```python
from build123d import *

# Parameters (mm, degrees)
SKETCH1_W               = 51
SKETCH1_H               = 26
PCB_DEPTH               = 1.6
MOUNT_HOLE_1_DEPTH      = 58.267442758
MOUNT_HOLE_1_DEPTH_BACK = 58.267442758
SKETCH2_R               = 1.5
MOUNT_HOLE_2_DEPTH      = 58.267442758
MOUNT_HOLE_2_DEPTH_BACK = 58.267442758
SKETCH3_R               = 1.5
MOUNT_HOLE_3_DEPTH      = 58.267442758
MOUNT_HOLE_3_DEPTH_BACK = 58.267442758
SKETCH4_R               = 1.5
MOUNT_HOLE_4_DEPTH      = 58.267442758
MOUNT_HOLE_4_DEPTH_BACK = 58.267442758
SKETCH5_R               = 1.5
INDUCTOR_START          = 1.6
SKETCH6_W               = 14
SKETCH6_H               = 14
INDUCTOR_DEPTH          = 8
CAP_IN_START            = 1.6
SKETCH7_R               = 5
CAP_IN_DEPTH            = 13
CAP_OUT_START           = 1.6
SKETCH8_R               = 5
CAP_OUT_DEPTH           = 13
HEATSINK_START          = 1.6
SKETCH9_W               = 8
SKETCH9_H               = 16
HEATSINK_DEPTH          = 11
TRIM_POT_START          = 1.6
SKETCH10_W              = 9.5
SKETCH10_H              = 4.5
TRIM_POT_DEPTH          = 9.5


with BuildPart() as part:
    # Sketch1 → PCB (new body)
    with BuildSketch(Plane(origin=(0, 0, 0), x_dir=(1, 0, 0), z_dir=(0, 1, 0))):
        with Locations((25.5, 13)):
            Rectangle(SKETCH1_W, SKETCH1_H)
    extrude(amount=PCB_DEPTH)

    # Sketch2 → Mount_hole_1 (cut, two sides: drawn at the far end of the back side and taken through both)
    with BuildSketch(Plane(origin=(0, 0, 0), x_dir=(1, 0, 0), z_dir=(0, 1, 0)).offset(-MOUNT_HOLE_1_DEPTH_BACK)):
        with Locations(Location((2.5, 2.5, 0), (0, 0, 270))):
            Circle(SKETCH2_R)
    extrude(amount=MOUNT_HOLE_1_DEPTH + MOUNT_HOLE_1_DEPTH_BACK, mode=Mode.SUBTRACT)

    # Sketch3 → Mount_hole_2 (cut, two sides: drawn at the far end of the back side and taken through both)
    with BuildSketch(Plane(origin=(0, 0, 0), x_dir=(1, 0, 0), z_dir=(0, 1, 0)).offset(-MOUNT_HOLE_2_DEPTH_BACK)):
        with Locations(Location((48.5, 2.5, 0), (0, 0, 270))):
            Circle(SKETCH3_R)
    extrude(amount=MOUNT_HOLE_2_DEPTH + MOUNT_HOLE_2_DEPTH_BACK, mode=Mode.SUBTRACT)

    # Sketch4 → Mount_hole_3 (cut, two sides: drawn at the far end of the back side and taken through both)
    with BuildSketch(Plane(origin=(0, 0, 0), x_dir=(1, 0, 0), z_dir=(0, 1, 0)).offset(-MOUNT_HOLE_3_DEPTH_BACK)):
        with Locations(Location((2.5, 23.5, 0), (0, 0, 270))):
            Circle(SKETCH4_R)
    extrude(amount=MOUNT_HOLE_3_DEPTH + MOUNT_HOLE_3_DEPTH_BACK, mode=Mode.SUBTRACT)

    # Sketch5 → Mount_hole_4 (cut, two sides: drawn at the far end of the back side and taken through both)
    with BuildSketch(Plane(origin=(0, 0, 0), x_dir=(1, 0, 0), z_dir=(0, 1, 0)).offset(-MOUNT_HOLE_4_DEPTH_BACK)):
        with Locations(Location((48.5, 23.5, 0), (0, 0, 270))):
            Circle(SKETCH5_R)
    extrude(amount=MOUNT_HOLE_4_DEPTH + MOUNT_HOLE_4_DEPTH_BACK, mode=Mode.SUBTRACT)

    # Sketch6 → Inductor (add)
    with BuildSketch(Plane(origin=(0, 0, 0), x_dir=(1, 0, 0), z_dir=(0, 1, 0)).offset(INDUCTOR_START)):
        with Locations((21, 13)):
            Rectangle(SKETCH6_W, SKETCH6_H)
    extrude(amount=INDUCTOR_DEPTH)

    # Sketch7 → Cap_in (add)
    with BuildSketch(Plane(origin=(0, 0, 0), x_dir=(1, 0, 0), z_dir=(0, 1, 0)).offset(CAP_IN_START)):
        with Locations(Location((7, 13, 0), (0, 0, 90))):
            Circle(SKETCH7_R)
    extrude(amount=CAP_IN_DEPTH)

    # Sketch8 → Cap_out (add)
    with BuildSketch(Plane(origin=(0, 0, 0), x_dir=(1, 0, 0), z_dir=(0, 1, 0)).offset(CAP_OUT_START)):
        with Locations(Location((44, 13, 0), (0, 0, 90))):
            Circle(SKETCH8_R)
    extrude(amount=CAP_OUT_DEPTH)

    # Sketch9 → Heatsink (add)
    with BuildSketch(Plane(origin=(0, 0, 0), x_dir=(1, 0, 0), z_dir=(0, 1, 0)).offset(HEATSINK_START)):
        with Locations((32.5, 13)):
            Rectangle(SKETCH9_W, SKETCH9_H)
    extrude(amount=HEATSINK_DEPTH)

    # Sketch10 → Trim_pot (add)
    with BuildSketch(Plane(origin=(0, 0, 0), x_dir=(1, 0, 0), z_dir=(0, 1, 0)).offset(TRIM_POT_START)):
        with Locations((34.75, 2.75)):
            Rectangle(SKETCH10_W, SKETCH10_H)
    extrude(amount=TRIM_POT_DEPTH)


solid = part.part
```
The model under review builds one solid part; all positions refer to its coordinate system, in mm. A direction names the side the tool comes from. Give positions to 0.01 mm unless a question says otherwise; leave off trailing zeros. Loops run counter-clockwise (first coordinate to the right, second up) from the corner with the lowest first, then second, coordinate; pieces in that order, holes last. Notation, with made-up numbers: (-23, 64.25) -> (2, 64.25) arc R13 cw to (2, 80.25) -> close; hole circle Ø7 at (-2.5, -21.5). An arc over 180 degrees is marked (long way). Use CSV: the item, a comma, the result in double quotes.
1. For P1, Ø5, axis at x = 48.5, z = -2.5, coming from the +Y side; P2, Ø5, axis at y = 8, z = -3, coming from the +X side; P3, Ø4, axis at x = 33.5, y = 5, coming from the +Z side; P4, Ø1.5, axis at x = 13, y = 3.5, coming from the -Z side, all flat-tipped, find the tip position at first contact; note any pin that passes through.
Result:
P1,"stops at y = 1.6"
P2,"stops at x = 39.5"
P3,"stops at z = -0.5"
P4,"passes through"
2. To check wall thickness, follow probe 1 along X at (y, z) = (0.4, -23.5); probe 2 along Z at (x, y) = (48.5, 1.05); probe 3 along X at (y, z) = (10.5, -13). State the ranges of each line that lie inside material, in increasing order. Write a range as from..to.
Result:
probe 1,"x = 0..1, 4..47, 50..51"
probe 2,"z = -26..-25, -22..-4, -1..0"
probe 3,"x = 2..12, 28.5..36.5, 39..49"
3. Consider section D-D, the plane z = -4.5. Write out the cut boundary in (x, y).
Result:
outline,"(0, 0) -> (51, 0) -> (51, 1.6) -> (39.5, 1.6) -> (39.5, 11.1) -> (30, 11.1) -> (30, 1.6) -> (0, 1.6) -> close"
4. The part is to be moulded in two halves that separate along Z. For faces 5 (the face through (35, 6, -0.5)), 6 (the face through (21, 6, -20)), 7 (the face through (1.17, 0.79, -1.81)), 8 (the face through (44, 14.6, -13)), say which applies: +Z half, -Z half, draft (parallel to the pull), parting line (faces both ways), or undercut.
Result:
face 5,"+Z half"
face 6,"-Z half"
face 7,"undercut"
face 8,"draft"
5. Consider section B-B, the plane y = 7.5. Write out the cut boundary in (x, z), then the cut area to 3 significant figures.
Result:
outline,"circle Ø10 at (7, -13); (14, -20) -> (28, -20) -> (28, -6) -> (14, -6) -> close; (28.5, -21) -> (36.5, -21) -> (36.5, -5) -> (39.5, -5) -> (39.5, -0.5) -> (30, -0.5) -> (30, -5) -> (28.5, -5) -> close; circle Ø10 at (44, -13)"
area,"524 mm²"
6. Consider section A-A, the plane z = -23.5. Write out the cut boundary in (x, y), then the cut area to 3 significant figures.
Result:
outline,"(0, 0) -> (1, 0) -> (1, 1.6) -> (0, 1.6) -> close; (4, 0) -> (47, 0) -> (47, 1.6) -> (4, 1.6) -> close; (50, 0) -> (51, 0) -> (51, 1.6) -> (50, 1.6) -> close"
area,"72.0 mm²"
7. Machinability: for faces 1 (the face through (35, 11.1, -3)), 2 (the face through (25, 0, -13)), 3 (the face through (39.5, 6, -3)), 4 (the face through (21, 9.6, -13)), which of the approach directions +Z, -Z, +X, -X, +Y, -Y give a long, thin tool a straight path to every point of the face, cutting with its end or side? Answer none if there is none.
Result:
face 1,"+Z, +X, -X, +Y"
face 2,"+Z, -Z, +X, -X, -Y"
face 3,"+Z, +X, +Y"
face 4,"+Z, -Z, +Y"
8. Consider section C-C, the plane x = 29. Write out the cut boundary in (y, z), then the cut area to 3 significant figures.
Result:
outline,"(0, -26) -> (1.6, -26) -> (1.6, -21) -> (12.6, -21) -> (12.6, -5) -> (1.6, -5) -> (1.6, 0) -> (0, 0) -> close"
area,"218 mm²"
